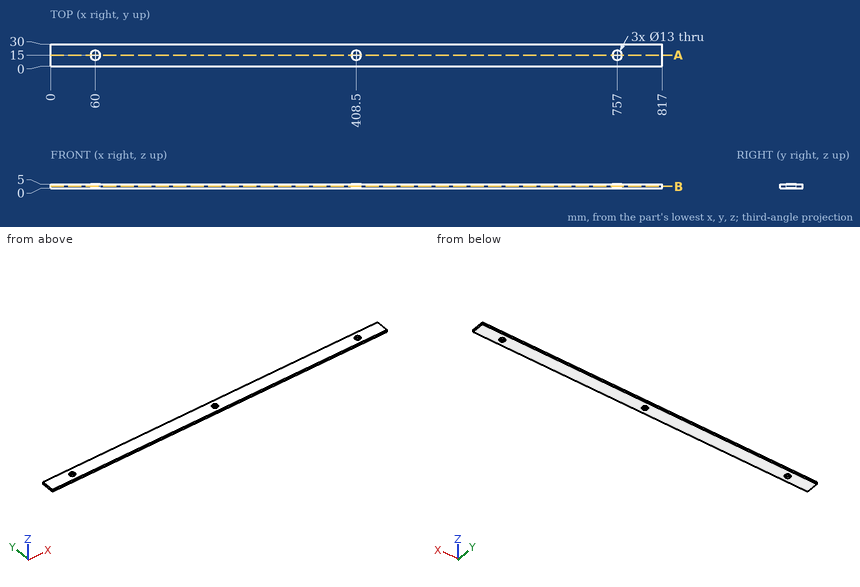
Check sheet for the drawn part. Datum: minimum x, y, z corner. Units: mm. Round coordinates to 2 decimals unless told otherwise and drop trailing zeros. Loops run counter-clockwise (first coordinate to the right, second up) from the corner with the lowest first, then second, coordinate; pieces in that order, holes last. Notation, with made-up numbers: (-7.5, 12) - (47.5, 12) arc R24 ccw to (47.5, 33) - close; hole circle Ø10 at (-9, -3). An arc over 180 degrees is marked (long way). Write each question's results on one line, items separated by ' | '. Start each with the question number.
Q1. Cross-section at A-A on y = 15. Enter the section's corners in (x, z).
Q2. Cross-section at B-B on z = 2.4. Enter the section's corners in (x, y).
Q3. Thickness scan on line 1 (X direction, y = 14.5, z = 3.85); line 2 (X direction, y = 14, z = 4.75); line 3 (Y direction, x = 60, z = 3.05). Record the ranges inside material, lowest first. Write a range as [from, to].
Answers below:
1) outline: (0, 0) - (53.5, 0) - (53.5, 5) - (0, 5) - close; (66.5, 0) - (402, 0) - (402, 5) - (66.5, 5) - close; (415, 0) - (750.5, 0) - (750.5, 5) - (415, 5) - close; (763.5, 0) - (817, 0) - (817, 5) - (763.5, 5) - close
2) outline: (0, 0) - (817, 0) - (817, 30) - (0, 30) - close; hole circle Ø13 at (60, 15); hole circle Ø13 at (408.5, 15); hole circle Ø13 at (757, 15)
3) line 1: x = [0, 53.52], [66.48, 402.02], [414.98, 750.52], [763.48, 817] | line 2: x = [0, 53.58], [66.42, 402.08], [414.92, 750.58], [763.42, 817] | line 3: y = [0, 8.5], [21.5, 30]
